from build123d import *

# Parameters (mm, degrees)
BOSS_EXTRUDE1_DEPTH = 65
SKETCH2_R           = 2
M_DRILL_DEPTH       = 20
SKETCH3_R           = 2.25
M4_THROUGH_DEPTH    = 8
CHAMFER1_SIZE       = 2


with BuildPart() as part:
    # Sketch1 → Boss-Extrude1 (new body)
    with BuildSketch(Plane(origin=(0, 0, 0), x_dir=(0, 0, -1), z_dir=(1, 0, 0))):
        Polygon((0, 0), (0, 19), (7.56469212, 19), (5, 13.5), (22.56469212, 13.5), (20, 8), (55, 8), (55, 0), align=None)
    extrude(amount=BOSS_EXTRUDE1_DEPTH)

    # Sketch2 → M$_DRILL (cut)
    with BuildSketch(Plane(origin=(0, 0, -55), x_dir=(-1, 0, 0), z_dir=(0, 0, -1))):
        with Locations((-12.5, 4.5)):
            Circle(SKETCH2_R)
        with Locations(Location((-52.5, 4.5, 0), (0, 0, 180))):
            Circle(SKETCH2_R)
    extrude(amount=-M_DRILL_DEPTH, mode=Mode.SUBTRACT)

    # Sketch3 → M4_through (cut)
    with BuildSketch(Plane(origin=(0, 8, 0), x_dir=(1, 0, 0), z_dir=(0, 1, 0))):
        with Locations(Location((39.5, 42, 0), (0, 0, 270))):
            Circle(SKETCH3_R)
        with Locations(Location((29, 35.937822174, 0), (0, 0, 270))):
            Circle(SKETCH3_R)
        with Locations(Location((29, 48.062177826, 0), (0, 0, 270))):
            Circle(SKETCH3_R)
    extrude(amount=-M4_THROUGH_DEPTH, mode=Mode.SUBTRACT)

    # Chamfer1
    chamfer1_edges = [part.edges().sort_by_distance(p)[0] for p in [
        (39.5, 8, -44.25),
        (29, 8, -38.187822174),
        (29, 8, -50.312177826),
    ]]
    chamfer(chamfer1_edges, length=CHAMFER1_SIZE)


solid = part.part
Verification items for the finished model (mm, model axes). A direction names the side the tool comes from. Give positions to 0.01 mm unless a question says otherwise; leave off trailing zeros. Loops run counter-clockwise (first coordinate to the right, second up) from the corner with the lowest first, then second, coordinate; pieces in that order, holes last.
1) Set-up check for faces 1 (the flat face through (32.04, 16.29, -6.3)), 2 (the cylindrical face through (14.1, 3.3, -45.1)), 3 (the cylindrical face through (41.73, 3.04, -42.29)): record each of +Z, -Z, +X, -X, +Y, -Y from which the full face is reachable in a straight line by a thin tool's end or side.
2) Sectioned sample at A-A, the plane z = -42. Enter the section's corners in (x, y).
3) Sectioned sample at C-C, the plane x = 29. Enter the section's corners in (y, z).
4) Sectioned sample at B-B, the plane y = 4.5. Enter the section's corners in (x, z).
5) Draft check along Z on faces 4 (the flat face through (32, 0, -28)), 5 (the flat face through (32, 4, -55)), 6 (the conical face through (28.09, 6.125, -45.868)), 7 (the cylindrical face through (29.1, 3.04, -50.31)). Enter one of: pulls with the +Z half, pulls with the -Z half, needs draft (parallel to the pull), parting line crosses it, or undercut.
6) Depth check by flat-ended pin: pin 1 Ø3.5 at (x, y) = (12.5, 4.5) entering from -Z; pin 2 Ø3.5 at (x, z) = (39.5, -42) entering from +Y; pin 3 Ø10.5 at (x, z) = (19, -32.5) entering from +Y. Enter the tip coordinate at first touch or a pass-through.
7) Thickness scan on line 1 along X through (y, z) = (4.4, -42); line 2 along X through (y, z) = (1.5, -42); line 3 along Y through (x, z) = (52.5, -47.5). Record the ranges inside material, lowest first.
8) Sectioned sample at D-D, the plane x = 39.5. Enter the section's corners in (y, z), then the cut area to 3 significant figures.
Answers:
1. face 1: -Z, +X, -X
1. face 2: -Z
1. face 3: +Y, -Y
2. outline: (0, 0) - (37.25, 0) - (37.25, 6) - (35.25, 8) - (0, 8) - close; (41.75, 0) - (65, 0) - (65, 8) - (43.75, 8) - (41.75, 6) - close; hole circle Ø4 at (12.5, 4.5); hole circle Ø4 at (52.5, 4.5)
3. outline: (0, -55) - (8, -55) - (8, -52.31) - (6, -50.31) - (0, -50.31) - close; (0, -45.81) - (6, -45.81) - (8, -43.81) - (8, -40.19) - (6, -38.19) - (0, -38.19) - close; (0, -33.69) - (6, -33.69) - (8, -31.69) - (8, -20) - (13.5, -22.56) - (13.5, -5) - (19, -7.56) - (19, 0) - (0, 0) - close
4. outline: (0, -55) - (10.5, -55) - (10.5, -35) - (14.5, -35) - (14.5, -55) - (50.5, -55) - (50.5, -35) - (54.5, -35) - (54.5, -55) - (65, -55) - (65, 0) - (0, 0) - close; hole circle Ø4.5 at (29, -48.06); hole circle Ø4.5 at (29, -35.94); hole circle Ø4.5 at (39.5, -42)
5. face 4: needs draft
5. face 5: pulls with the -Z half
5. face 6: undercut
5. face 7: undercut
6. pin 1: stops at z = -35
6. pin 2: passes through
6. pin 3: stops at y = 8
7. line 1: x = 0 to 10.5, 14.5 to 37.25, 41.75 to 50.5, 54.5 to 65
7. line 2: x = 0 to 37.25, 41.75 to 65
7. line 3: y = 0 to 2.5, 6.5 to 8
8. outline: (0, -55) - (8, -55) - (8, -46.25) - (6, -44.25) - (0, -44.25) - close; (0, -39.75) - (6, -39.75) - (8, -37.75) - (8, -20) - (13.5, -22.56) - (13.5, -5) - (19, -7.56) - (19, 0) - (0, 0) - close
8. area: 552 mm2
